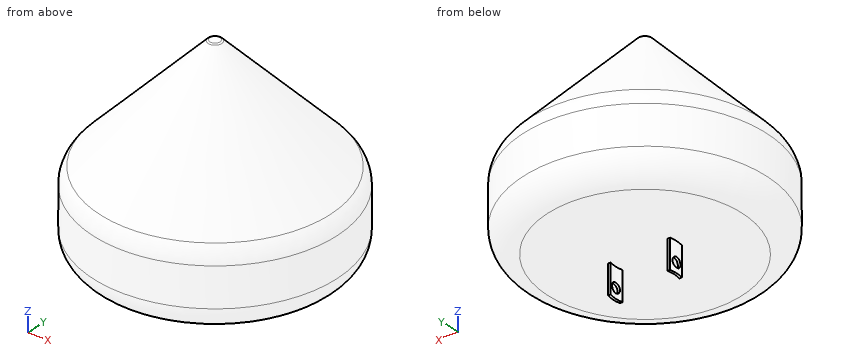
```python
from build123d import *

# Parameters (mm, degrees)
SKETCH2_R               = 50
BOSS_EXTRUDE1_DEPTH     = 30
SKETCH4_R               = 2.5
FILLET1_R               = 10
FILLET3_R               = 1
SKETCH6_R               = 13
BOSS_EXTRUDE2_DEPTH     = 12
SKETCH7_R               = 12
CUT_EXTRUDE1_DEPTH      = 12
SKETCH8_R               = 2
CUT_EXTRUDE2_DEPTH      = 20
CUT_EXTRUDE2_DEPTH_BACK = 19
SKETCH9_W               = 12
SKETCH9_H               = 10
CUT_EXTRUDE3_DEPTH      = 17
CUT_EXTRUDE3_DEPTH_BACK = 23
FILLET4_R               = 10


with BuildPart() as part:
    # Sketch2 → Boss-Extrude1 (new body)
    with BuildSketch(Plane.XY):
        Circle(SKETCH2_R)
    extrude(amount=BOSS_EXTRUDE1_DEPTH)

    # Sketch4 → section 1 of loft2
    with BuildSketch(Plane.XY.offset(80), mode=Mode.PRIVATE) as loft2_s1:
        Circle(SKETCH4_R)
    # loft up to a face of the part (loft2)
    loft([Face(Wire([part.edges().sort_by_distance((-34.227355296, 36.448431371, 30))[0]])), loft2_s1.sketch])

    # Fillet1
    fillet1_edges = [part.edges().sort_by_distance(p)[0] for p in [
        (-50, 0, 30),
    ]]
    fillet(fillet1_edges, radius=FILLET1_R)

    # Fillet3
    fillet3_edges = [part.edges().sort_by_distance(p)[0] for p in [
        (-2.5, 0, 80),
    ]]
    fillet(fillet3_edges, radius=FILLET3_R)

    # Sketch6 → Boss-Extrude2 (add)
    with BuildSketch(Plane(origin=(0, 0, 0), x_dir=(-1, 0, 0), z_dir=(0, 0, -1))):
        Circle(SKETCH6_R)
    extrude(amount=BOSS_EXTRUDE2_DEPTH)

    # Sketch7 → Cut-Extrude1 (cut)
    with BuildSketch(Plane(origin=(0, 0, -12), x_dir=(-1, 0, 0), z_dir=(0, 0, -1))):
        Circle(SKETCH7_R)
    extrude(amount=-CUT_EXTRUDE1_DEPTH, mode=Mode.SUBTRACT)

    # Sketch8 → Cut-Extrude2 (cut, two sides)
    with BuildSketch(Plane(origin=(0, 0, 0), x_dir=(0, 0, -1), z_dir=(1, 0, 0))) as cut_extrude2_sk:
        with Locations(Location((7.94, 0, 0), (0, 0, 180))):
            Circle(SKETCH8_R)
    extrude(amount=CUT_EXTRUDE2_DEPTH, mode=Mode.SUBTRACT)
    extrude(cut_extrude2_sk.sketch, amount=-CUT_EXTRUDE2_DEPTH_BACK, mode=Mode.SUBTRACT)

    # Sketch9 → Cut-Extrude3 (cut, two sides)
    with BuildSketch(Plane(origin=(0, 0, 0), x_dir=(0, 0, -1), z_dir=(1, 0, 0))) as cut_extrude3_sk:
        with Locations((6, 8)):
            Rectangle(SKETCH9_W, SKETCH9_H)
        with Locations((6, -8)):
            Rectangle(SKETCH9_W, SKETCH9_H)
    extrude(amount=CUT_EXTRUDE3_DEPTH, mode=Mode.SUBTRACT)
    extrude(cut_extrude3_sk.sketch, amount=-CUT_EXTRUDE3_DEPTH_BACK, mode=Mode.SUBTRACT)

    # Fillet4
    fillet4_edges = [part.edges().sort_by_distance(p)[0] for p in [
        (-50, 0, 0),
    ]]
    fillet(fillet4_edges, radius=FILLET4_R)


solid = part.part
```
Geometry: final body of the model. Coordinates: model frame, mm. Round coordinates to 2 decimals unless told otherwise and drop trailing zeros. Write each loop counter-clockwise with the first axis right and the second up, starting at its lowest first coordinate (ties: lowest second). Pieces come first, ordered by that corner, then holes. Notation, with made-up numbers: M 72,39 L 124,39 A21 cw 124,52 Z; hole C 49,-5 d4. An arc over 180 degrees is marked long. Answer in a Markdown table with one row per item. Add a question column.
(1) Ray query, L1, parallel to Y at x = 12.2, z = -7.94; L2, parallel to Y at x = 12, z = -7; L3, parallel to X at y = 5.5, z = 67. Return the intervals inside material, ascending.
(2) Cut plane A-A, the plane z = -7.94. Return the cut outline in (x, y), then the cut area to 3 significant figures.
(3) Cut plane C-C, the plane z = 53. Return the cut outline in (x, y), then the cut area to 3 significant figures.
(4) Contact query for flat-ended pins moving along their axis: pin 1 (3 mm diameter, centred on x = -5.5, z = 65, fed in from -Y); pin 2 (12 mm diameter, centred on x = -10.5, z = 6.5, fed in from -Y); pin 3 (12 mm diameter, centred on x = -8.5, z = 24.5, fed in from -Y). Output: stop coordinate, or through.
(5) Cut plane B-B, the plane z = 41. Return the cut outline in (x, y), then the cut area to 3 significant figures.
Established:
| question | item | result |
|---|---|---|
| 1 | L1 | -3 to -2, 2 to 3 |
| 1 | L2 | -3 to -1.77, 1.77 to 3 |
| 1 | L3 | -13.79 to 13.79 |
| 2 | outline | M -12.85,-2 A13 ccw -12.65,-3 L -11.62,-3 A12 cw -11.83,-2 Z; M -12.85,2 L -11.83,2 A12 cw -11.62,3 L -12.65,3 A13 ccw Z; M 11.62,-3 L 12.65,-3 A13 ccw 12.85,-2 L 11.83,-2 A12 cw Z; M 11.62,3 A12 cw 11.83,2 L 12.85,2 A13 ccw 12.65,3 Z |
| 2 | area | 4.08 mm² |
| 3 | outline | C 0,0 d56.3 |
| 3 | area | 2,490 mm² |
| 4 | pin 1 | y = -17.39 |
| 4 | pin 2 | y = -49.71 |
| 4 | pin 3 | y = -49.94 |
| 5 | outline | C 0,0 d79.1 |
| 5 | area | 4,910 mm² |
